For this review, take the finished solid that the model builds, in its own axes (mm). A direction names the side the tool comes from. Give positions to 0.01 mm unless a question says otherwise; leave off trailing zeros. Order: outer loops, then holes, each group sorted by start corner. A loop starts at its lowest first (then second) coordinate and runs counter-clockwise, first axis right, second up. Notation, with made-up numbers: M -31.75,3 L -22.75,3 A31 ccw -22.75,41 Z; hole C -33,63.25 d11. An arc over 180 degrees is marked long. Answer as CSV lines item,"result". Start each with the question number.
1. We need section C-C, the plane z = 7.25. Give the boundary of the cut face in (x, y).
2. Machinability: for faces 1 (the conical face through (3.5, -0.78, 12.76)), 2 (the flat face through (-0.1, -5.5, 5.5)), which of the approach directions +Z, -Z, +X, -X, +Y, -Y give a long, thin tool a straight path to every point of the face, cutting with its end or side? Answer none if there is none.
3. We need section B-B, the plane z = 3.25. Give the boundary of the cut face in (x, y).
4. Clearance check with flat-ended pins moving along their axes: P1, Ø2, axis at x = -4, y = -1, coming from the +Z side; P2, Ø1.5, axis at x = 3, z = 7, coming from the +Y side; P3, Ø4.5, axis at x = -1, y = -1, coming from the -Z side. State where each tip first meets the part, or that it passes through.
5. Mouldability with a two-part tool opening along Y and no side actions: class faces 3 (the flat face through (1.3, 1.3, 13)), 4 (the cylindrical face through (-0.66, -14.985, 4.102)), 5 (the flat face through (0, 6, 2)), 6 (the flat face through (-2.685, 0, 7)) as pulls with the +Y half, pulls with the -Y half, needs draft (parallel to the pull), parting line crosses it, or undercut.
6. We need section A-A, the plane y = 0. Give the boundary of the cut face in (x, z), and give its area (3 significant figures).
7. For line 1 along X through (y, z) = (0, 10.75); line 2 along Y through (x, z) = (-4.5, 1.5); line 3 along Y through (x, z) = (10.75, 5), list the stretches that pass through material, from the lowest coordinate up.
from build123d import *

# Parameters (mm, degrees)
SKETCH_W        = 12
SKETCH_H        = 12
POCKET_DEPTH    = 6
POCKET001_DEPTH = 3
CHAMFER_SIZE    = 1
CHAMFER001_SIZE = 1


with BuildPart() as part:
    # Sketch002 → Revolution (revolve)
    with BuildSketch(Plane.YZ):
        Polygon((1.6, 13), (1.6, 0), (15, 0), (15, 8.09067), (3, 13), align=None)
    revolve(axis=Axis((0, 0, 0), (0, 0, 1)))

    # Sketch (on Face2 of Revolution) → Pocket (cut)
    with BuildSketch(Plane.YX):
        Rectangle(SKETCH_W, SKETCH_H)
    extrude(amount=-POCKET_DEPTH, mode=Mode.SUBTRACT)

    # Sketch003 (on Face2 of Pocket) → Pocket001 (cut)
    with BuildSketch(Plane.YX.offset(-6)):
        Polygon((3.1, 0), (1.55, 2.684679), (-1.55, 2.684679), (-3.1, 0), (-1.55, -2.684679), (1.55, -2.684679), align=None)
    extrude(amount=-POCKET001_DEPTH, mode=Mode.SUBTRACT)

    # Chamfer
    chamfer_edges = [part.edges().sort_by_distance(p)[0] for p in [
        (0, -6, 6),
        (0, 6, 6),
        (-6, 0, 6),
        (6, 0, 6),
    ]]
    chamfer(chamfer_edges, length=CHAMFER_SIZE)

    # Chamfer001
    chamfer001_edges = [part.edges().sort_by_distance(p)[0] for p in [
        (0, -1.6, 9),
    ]]
    chamfer(chamfer001_edges, length=CHAMFER001_SIZE)


solid = part.part
Result set:
1,outline,"C 0,0 d30; hole M -2.68,-1.55 L 0,-3.1 L 2.68,-1.55 L 2.68,1.55 L 0,3.1 L -2.68,1.55 Z"
2,face 1,"+Z"
2,face 2,"-Z"
3,outline,"C 0,0 d30; hole M -6,-6 L 6,-6 L 6,6 L -6,6 Z"
4,P1,"z = 12.95"
4,P2,"y = 14.83"
4,P3,"z = 6"
5,face 3,"needs draft"
5,face 4,"parting line crosses it"
5,face 5,"undercut"
5,face 6,"undercut"
6,outline,"M -15,0 L -6,0 L -6,5 L -5,6 L -2.68,6 L -2.68,9 L -2.6,9 L -1.6,10 L -1.6,13 L -3,13 L -15,8.09 Z; M 1.6,10 L 2.6,9 L 2.68,9 L 2.68,6 L 5,6 L 6,5 L 6,0 L 15,0 L 15,8.09 L 3,13 L 1.6,13 Z"
6,area,"230 mm2"
7,line 1,"-8.5 to -1.6, 1.6 to 8.5"
7,line 2,"-14.31 to -6, 6 to 14.31"
7,line 3,"-10.46 to 10.46"
